Design review of the part built by this model. Coordinates are the model's own, in mm. A direction names the side the tool comes from. Give positions to 0.01 mm unless a question says otherwise; leave off trailing zeros. Order: outer loops, then holes, each group sorted by start corner. A loop starts at its lowest first (then second) coordinate and runs counter-clockwise, first axis right, second up. Notation, with made-up numbers: (56, -11.5) -> (66, -11.5) arc R19 ccw to (66, 0.5) -> close; hole circle Ø1 at (72.5, 13.25). An arc over 180 degrees is marked (long way). Use a Markdown table: item, result. Add a question column.
```python
from build123d import *

# Parameters (mm, degrees)
FILLET_1_R          = 0.2
CUT_EXTRUDE_1_DEPTH = 1.5
SKETCH_3_R          = 1.5
EXTRUDE_1_DEPTH     = 6
CHAMFER_1_SIZE      = 0.5


with BuildPart() as part:
    # 草图1 → 旋转1 (revolve)
    with BuildSketch(Plane.XY):
        with BuildLine():
            Line((0, 0), (0, 2))
            Line((0, 2), (1.3, 2))
            ThreePointArc((1.3, 2), (2.370691821, 1.250626571), (2.75, 0))
            Line((2.75, 0), (0, 0))
        make_face()
    revolve(axis=Axis((0, 0, 0), (0, 1, 0)))

    # 圆角1
    fillet_1_edges = [part.edges().sort_by_distance(p)[0] for p in [
        (-2.75, 0, 0),
    ]]
    fillet(fillet_1_edges, radius=FILLET_1_R)

    # 草图2 → 切除-拉伸1 (cut)
    with BuildSketch(Plane(origin=(0, 2, 0), x_dir=(1, 0, 0), z_dir=(0, 1, 0))):
        Polygon((1.327905619, 0), (0.66395281, 1.15), (-0.66395281, 1.15), (-1.327905619, 0), (-0.66395281, -1.15), (0.66395281, -1.15), align=None)
    extrude(amount=-CUT_EXTRUDE_1_DEPTH, mode=Mode.SUBTRACT)

    # 草图3 → 凸台-拉伸1 (add)
    with BuildSketch(Plane.XZ):
        Circle(SKETCH_3_R)
    extrude(amount=EXTRUDE_1_DEPTH)

    # 倒角1
    chamfer_1_edges = [part.edges().sort_by_distance(p)[0] for p in [
        (-1.5, -6, 0),
    ]]
    chamfer(chamfer_1_edges, length=CHAMFER_1_SIZE)


solid = part.part
```
1) For L1, parallel to X at y = 1, z = -0.6; L2, parallel to Y at x = 2.5, z = 0.35; L3, parallel to X at y = 1, z = 0.95, list the stretches that pass through material, from the lowest coordinate up. Write a range as [from, to].
2) The part is to be moulded in two halves that separate along X. For faces 1 (the flat face through (0, -6, 0)), 2 (the flat face through (1, 1.26, -0.57)), 3 (the cylindrical face through (-1.5, -2.71, 0.07)), say which applies: +X half, -X half, draft (parallel to the pull), parting line (faces both ways), or undercut.
3) Machinability: for faces 4 (the flat face through (-0.991, 1.26, -0.583)), 5 (the flat face through (0, 0, 2)), which of the approach directions +Z, -Z, +X, -X, +Y, -Y give a long, thin tool a straight path to every point of the face, cutting with its end or side? Answer none if there is none.
4) Insertion check: pin 1 (1 mm diameter, centred on x = 1, z = 1.5, fed in from -Y); pin 2 (1 mm diameter, centred on x = -0.5, y = -1.5, fed in from +Z); pin 3 (1.5 mm diameter, centred on y = -2, z = 1, fed in from +X). Each pin has a flat end and moves straight along its axis. Give the tip position at first contact, or say it passes through.
5) Add section A-A (y = -1.5). Give the boundary of the cut face in (x, z).
Worked answers:
| question | item | result |
|---|---|---|
| 1 | L1 | [-2.45, -0.98], [0.98, 2.45] |
| 1 | L2 | [0, 1] |
| 1 | L3 | [-2.34, -0.78], [0.78, 2.34] |
| 2 | face 1 | draft |
| 2 | face 2 | undercut |
| 2 | face 3 | parting line |
| 3 | face 4 | +Y |
| 3 | face 5 | -Y |
| 4 | pin 1 | y = -5.7 |
| 4 | pin 2 | z = 1.5 |
| 4 | pin 3 | x = 1.48 |
| 5 | outline | circle Ø3 at (0, 0) |
